Check sheet for the modelled part. Datum: model origin and axes. Units: mm. A direction names the side the tool comes from. Coordinates: 2 decimals unless noted, no trailing zeros. Write each loop counter-clockwise with the first axis right and the second up, starting at its lowest first coordinate (ties: lowest second). Pieces come first, ordered by that corner, then holes. Notation, with made-up numbers: (6.5, -5.75) -> (30.5, -5.75) arc R21 ccw to (30.5, 27.25) -> close; hole circle Ø10 at (22, -9.5). An arc over 180 degrees is marked (long way). One line per item, written item: value. Start each with the question number.
1) Set-up check for faces 1 (the cylindrical face through (-58.77, 0.78, 12.19)), 2 (the flat face through (-19.05, 1, 16)): record each of +Z, -Z, +X, -X, +Y, -Y from which the full face is reachable in a straight line by a thin tool's end or side.
2) Gauge pin test, flat ends, axial feed: P1, Ø0.7, axis at y = 0.5, z = 21, coming from the +X side; P2, Ø0.9, axis at y = 1, z = 18, coming from the +X side; P3, Ø0.5, axis at x = -40.5, y = 1, coming from the +Z side. Record the tip position at first contact, or that the pin passes through.
3) Sectioned sample at A-A on y = 0.6. Enter the section's corners in (x, z), plus the area to 3 significant figures.
4) Draft check along X on faces 3 (the flat face through (-12.7, 1, 14)), 4 (the cylindrical face through (-17.35, 0.78, 6.28)), 5 (the flat face through (-22, 1, 16.693)). Enter one of: +X half, -X half, draft (parallel to the pull), parting line (faces both ways), or undercut.
5) Sectioned sample at D-D on x = -9. Enter the section's corners in (y, z).
6) Sectioned sample at B-B on z = 6.35. Enter the section's corners in (x, y).
7) Sectioned sample at C-C on x = -22. Enter the section's corners in (y, z), plus the area to 3 significant figures.
8) Scan lines: line 1 along Z through (x, y) = (-52.5, 0.4); line 2 along Z through (x, y) = (-38.5, 0.7); line 3 along X through (y, z) = (0.9, 18.25). Record each from-to range of solid material in increasing order. Write a range as [from, to].
Autodesk Inventor part; units mm, degrees
ref_plane "YZ Plane" through (0, 0, 0) normal (1, 0, 0) x (0, 1, 0)
ref_plane "XZ Plane" through (0, 0, 0) normal (0, 1, 0) x (-1, 0, 0)
ref_plane "XY Plane" through (0, 0, 0) normal (0, 0, 1) x (1, 0, 0)
sketch "Sketch1" plane through (0, 0, 0) normal (0, 1, 0) x (-1, 0, 0)
  line L0 (6.35, 11.0627) -> (0, 11.0627)
  line L1 (0, 11.0627) -> (0, 0)
  line L2 (0, 0) -> (76.2, 0)
  line L3 (6.35, 11.0627) -> (6.35, 12.2238)
  line L4 (6.35, 12.2238) -> (12.7, 12.2238)
  line L5 (12.7, 12.2238) -> (12.7, 14.8493)
  line L6 (12.7, 14.8493) -> (19.05, 14.8493)
  line L7 (19.05, 14.8493) -> (19.05, 16.6932)
  line L8 (19.05, 16.6932) -> (25.4, 16.6932)
  line L9 (25.4, 16.6932) -> (25.4, 17.9429)
  line L10 (25.4, 17.9429) -> (31.75, 17.9429)
  line L11 (31.75, 17.9429) -> (31.75, 18.7178)
  line L12 (31.75, 18.7178) -> (38.1, 18.7178)
  line L13 (38.1, 18.7178) -> (38.1, 19.7994)
  line L14 (38.1, 19.7994) -> (44.45, 19.7994)
  line L15 (44.45, 19.7994) -> (44.45, 20.4702)
  line L16 (44.45, 20.4702) -> (50.8, 20.4702)
  line L17 (50.8, 20.4702) -> (50.8, 21.1032)
  line L18 (50.8, 21.1032) -> (57.15, 21.1032)
  line L19 (57.15, 21.1032) -> (57.15, 21.4063)
  line L20 (57.15, 21.4063) -> (63.5, 21.4063)
  line L21 (63.5, 21.4063) -> (63.5, 21.9869)
  line L22 (63.5, 21.9869) -> (69.85, 21.9869)
  line L23 (69.85, 21.9869) -> (69.85, 22.5348)
  line L24 (69.85, 22.5348) -> (76.2, 22.5348)
  line L25 (76.2, 0) -> (76.2, 22.5348)
  circle A0 centre (19.05, 6.35) radius 1.7
  circle A1 centre (57.15, 12.7) radius 1.7
extrude "Extrusion1" add sketch "Sketch1" along normal blind 1.5875
properties part number "twinkle_twinkle_base"
Answers:
1. face 1: +Y, -Y
1. face 2: +Z, +X, +Y, -Y
2. P1: stops at x = -50.8
2. P2: stops at x = -25.4
2. P3: stops at z = 19.8
3. outline: (-76.2, 0) -> (0, 0) -> (0, 11.06) -> (-6.35, 11.06) -> (-6.35, 12.22) -> (-12.7, 12.22) -> (-12.7, 14.85) -> (-19.05, 14.85) -> (-19.05, 16.69) -> (-25.4, 16.69) -> (-25.4, 17.94) -> (-31.75, 17.94) -> (-31.75, 18.72) -> (-38.1, 18.72) -> (-38.1, 19.8) -> (-44.45, 19.8) -> (-44.45, 20.47) -> (-50.8, 20.47) -> (-50.8, 21.1) -> (-57.15, 21.1) -> (-57.15, 21.41) -> (-63.5, 21.41) -> (-63.5, 21.99) -> (-69.85, 21.99) -> (-69.85, 22.53) -> (-76.2, 22.53) -> close; hole circle Ø3.4 at (-57.15, 12.7); hole circle Ø3.4 at (-19.05, 6.35)
3. area: 1,370 mm2
4. face 3: +X half
4. face 4: undercut
4. face 5: draft
5. outline: (0, 0) -> (1.59, 0) -> (1.59, 12.22) -> (0, 12.22) -> close
6. outline: (-76.2, 0) -> (-20.75, 0) -> (-20.75, 1.59) -> (-76.2, 1.59) -> close; (-17.35, 0) -> (0, 0) -> (0, 1.59) -> (-17.35, 1.59) -> close
7. outline: (0, 0) -> (1.59, 0) -> (1.59, 16.69) -> (0, 16.69) -> close
7. area: 26.5 mm2
8. line 1: z = [0, 21.1]
8. line 2: z = [0, 19.8]
8. line 3: x = [-76.2, -31.75]
